Design review of the part built by this model. Coordinates are the model's own, in mm. Coordinates: 2 decimals unless noted, no trailing zeros. Write each loop counter-clockwise with the first axis right and the second up, starting at its lowest first coordinate (ties: lowest second). Pieces come first, ordered by that corner, then holes. Notation, with made-up numbers: (6, -9.75) -> (16, -9.75) arc R26 cw to (16, 25.25) -> close; hole circle Ø10 at (68.5, 42). An arc over 180 degrees is marked (long way). Return JSON: item names as keys, results as strings. Group by question number.
from build123d import *

# Parameters (mm, degrees)
SKETCH1_W           = 100
SKETCH1_H           = 100
SKETCH1_R           = 5
SKETCH1_R_2         = 3
BOSS_EXTRUDE1_DEPTH = 10


with BuildPart() as part:
    # Sketch1 → Boss-Extrude1 (new body)
    with BuildSketch(Plane(origin=(0, 0, 0), x_dir=(1, 0, 0), z_dir=(0, 1, 0))):
        Rectangle(SKETCH1_W, SKETCH1_H)
        with Locations(Location((0, 0, 0), (0, 0, 270))):
            Circle(SKETCH1_R, mode=Mode.SUBTRACT)
        with Locations(Location((-7.5, 35, 0), (0, 0, 270))):
            Circle(SKETCH1_R_2, mode=Mode.SUBTRACT)
        with Locations(Location((7.5, 35, 0), (0, 0, 270))):
            Circle(SKETCH1_R_2, mode=Mode.SUBTRACT)
        with Locations(Location((35, 7.5, 0), (0, 0, 270))):
            Circle(SKETCH1_R_2, mode=Mode.SUBTRACT)
        with Locations(Location((35, -7.5, 0), (0, 0, 270))):
            Circle(SKETCH1_R_2, mode=Mode.SUBTRACT)
        with Locations(Location((7.5, -35, 0), (0, 0, 270))):
            Circle(SKETCH1_R_2, mode=Mode.SUBTRACT)
        with Locations(Location((-7.5, -35, 0), (0, 0, 270))):
            Circle(SKETCH1_R_2, mode=Mode.SUBTRACT)
        with Locations(Location((-35, -7.5, 0), (0, 0, 270))):
            Circle(SKETCH1_R_2, mode=Mode.SUBTRACT)
        with Locations(Location((-35, 7.5, 0), (0, 0, 270))):
            Circle(SKETCH1_R_2, mode=Mode.SUBTRACT)
    extrude(amount=BOSS_EXTRUDE1_DEPTH)


solid = part.part
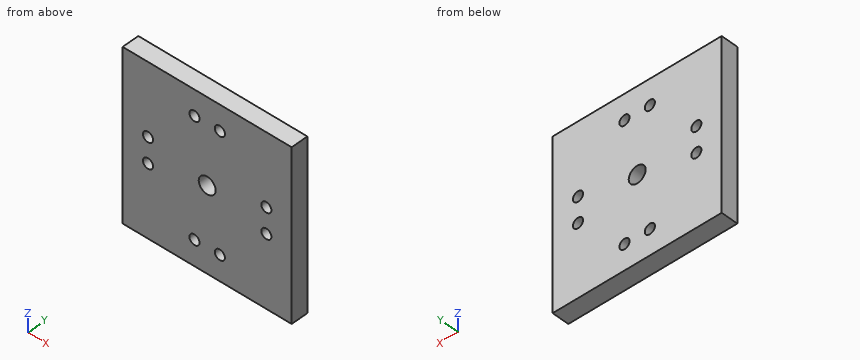
Q1. We need section C-C on y = 4.5. State how many separate pieces and enclosed holes the cut face has, plus the area to 3 significant figures.
Q2. We need section D-D on x = 35. Write out the cut boundary in (y, z), plus the area to 3 significant figures.
Q3. We need section B-B on x = 0. Write out the cut boundary in (y, z).
Q4. Wall thickness on L1, parallel to X at y = 7, z = 35; L2, parallel to X at y = 5.25, z = -7.5; L3, parallel to Z at x = 7, y = 1.5: over which ranges is each line inside the solid? List them lowest first.
Q5. For P1, Ø7, axis at x = 7.5, z = 35, coming from the +Y side, flat-tipped, find the tip position at first contact; note if it passes through.
Q6. We need section A-A on z = 7.5. Write out the cut boundary in (x, y), plus the area to 3 significant figures.
Findings below:
{
 "1": {"separate pieces": "1", "enclosed holes": "9", "area": "9,700 mm^2"},
 "2": {"outline": "(0, -50) -> (10, -50) -> (10, -10.5) -> (0, -10.5) -> close; (0, -4.5) -> (10, -4.5) -> (10, 4.5) -> (0, 4.5) -> close; (0, 10.5) -> (10, 10.5) -> (10, 50) -> (0, 50) -> close", "area": "880 mm^2"},
 "3": {"outline": "(0, -50) -> (10, -50) -> (10, -5) -> (0, -5) -> close; (0, 5) -> (10, 5) -> (10, 50) -> (0, 50) -> close"},
 "4": {"L1": "x = -50 to -10.5, -4.5 to 4.5, 10.5 to 50", "L2": "x = -50 to -38, -32 to 32, 38 to 50", "L3": "z = -50 to -37.96, -32.04 to 32.04, 37.96 to 50"},
 "5": {"P1": "stops at y = 10"},
 "6": {"outline": "(-50, 0) -> (-38, 0) -> (-38, 10) -> (-50, 10) -> close; (-32, 0) -> (32, 0) -> (32, 10) -> (-32, 10) -> close; (38, 0) -> (50, 0) -> (50, 10) -> (38, 10) -> close", "area": "880 mm^2"}
}
